Could you check a few things on this model? Use its own coordinates, in mm. A direction names the side the tool comes from. Coordinates: 2 decimals unless noted, no trailing zeros. Order: outer loops, then holes, each group sorted by start corner. A loop starts at its lowest first (then second) coordinate and runs counter-clockwise, first axis right, second up. Notation, with made-up numbers: (56.5, 16.25) - (109.5, 16.25) arc R19 cw to (109.5, 38.25) - close; hole circle Ø4 at (8, -33.75). An arc over 180 degrees is marked (long way). One line per item, written item: value. Start each with the question number.
from build123d import *

# Parameters (mm, degrees)
SKETCH1_W               = 28
SKETCH1_H               = 16
BOSS_EXTRUDE1_DEPTH     = 3
BOSS_EXTRU_1_DEPTH      = 5
BOSS_EXTRU_1_DEPTH_BACK = 18
ESQUISSE8_W             = 11.84
ESQUISSE8_H             = 2.37
ENL_V_MAT_EXTRU_4_DEPTH = 10
ESQUISSE9_W             = 22.6
ESQUISSE9_H             = 11.84
ENL_V_MAT_EXTRU_5_DEPTH = 1
ESQUISSE10_R            = 1.05
ENL_V_MAT_EXTRU_6_DEPTH = 52.879282956
CONG_3_R                = 1
CONG_4_R                = 5
CONG_5_R                = 2.5


with BuildPart() as part:
    # Sketch1 → Boss-Extrude1 (new body)
    with BuildSketch(Plane(origin=(0, 0, 0), x_dir=(1, 0, 0), z_dir=(0, 1, 0))):
        with Locations((14, 8)):
            Rectangle(SKETCH1_W, SKETCH1_H)
    extrude(amount=BOSS_EXTRUDE1_DEPTH)

    # Esquisse1 → Boss.-Extru.1 (add, two sides: drawn at the far end of the back side and taken through both)
    with BuildSketch(Plane.XY.offset(-BOSS_EXTRU_1_DEPTH_BACK)):
        Polygon((32.369048105, 3), (33.869048105, 3.9), (48.5, 3.9), (48.5, 0.9), (34.7, 0.9), (33.2, 0), (28, 0), (28, 3), align=None)
    extrude(amount=BOSS_EXTRU_1_DEPTH + BOSS_EXTRU_1_DEPTH_BACK)

    # Esquisse8 → Enlèv. mat.-Extru.4 (cut)
    with BuildSketch(Plane(origin=(0, 3.9, 0), x_dir=(1, 0, 0), z_dir=(0, 1, 0))):
        with Locations((41.52, 12.315)):
            Rectangle(ESQUISSE8_W, ESQUISSE8_H)
    extrude(amount=-ENL_V_MAT_EXTRU_4_DEPTH, mode=Mode.SUBTRACT)

    # Esquisse9 → Enlèv. mat.-Extru.5 (cut)
    with BuildSketch(Plane.XZ):
        with Locations((15.8, -8)):
            Rectangle(ESQUISSE9_W, ESQUISSE9_H)
    extrude(amount=-ENL_V_MAT_EXTRU_5_DEPTH, mode=Mode.SUBTRACT)

    # Esquisse10 → Enlèv. mat.-Extru.6 (cut, through all)
    with BuildSketch(Plane.XZ):
        with Locations(Location((31.11, 0, 0), (0, 0, 270))):
            Circle(ESQUISSE10_R)
        with Locations(Location((31.11, -16, 0), (0, 0, 270))):
            Circle(ESQUISSE10_R)
    extrude(amount=-ENL_V_MAT_EXTRU_6_DEPTH, mode=Mode.SUBTRACT)

    # Congé3
    cong_3_edges = [part.edges().sort_by_distance(p)[0] for p in [
        (28, 1.5, -16),
    ]]
    fillet(cong_3_edges, radius=CONG_3_R)
    cong_3_2_edges = [part.edges().sort_by_distance(p)[0] for p in [
        (28, 1.5, -18),
    ]]
    fillet(cong_3_2_edges, radius=CONG_3_R - 0.0001)  # a hair under: the kernel refuses the full size

    # Congé4
    cong_4_edges = [part.edges().sort_by_distance(p)[0] for p in [
        (48.5, 2.4, -18),
        (48.5, 2.4, 5),
        (0, 1.5, 0),
        (0, 1.5, -16),
    ]]
    fillet(cong_4_edges, radius=CONG_4_R)

    # Congé5
    cong_5_edges = [part.edges().sort_by_distance(p)[0] for p in [
        (28, 1.5, 0),
    ]]
    fillet(cong_5_edges, radius=CONG_5_R)
    cong_5_2_edges = [part.edges().sort_by_distance(p)[0] for p in [
        (28, 1.5, 5),
    ]]
    fillet(cong_5_2_edges, radius=CONG_5_R - 0.0001)  # a hair under: the kernel refuses the full size


solid = part.part
Q1. I want a section at A-A on x = 42. Please give me the cut outline in (y, z), then the cut area to 3 significant figures.
Q2. I want a section at C-C on z = -0.5. Please give me the cut outline in (x, y).
Q3. We'd pull the mould along Z, two halves only. Please class faces 1 (the flat face through (47.44, 2, -12)), 2 (the flat face through (37, 2, 5)), 3 (the cylindrical face through (2, 2, -15)), 4 (the cylindrical face through (32.15, 1.48, -15.86)): +Z half, -Z half, draft (parallel to the pull), parting line (faces both ways), or undercut.
Q4. I'm going to push flat-ended pins straight in: pin 1 (1 mm diameter, centred on x = 7.5, z = -9.5, fed in from -Y); pin 2 (6 mm diameter, centred on x = 10, z = -1, fed in from -Y); pin 3 (3 mm diameter, centred on x = 32, z = 1.5, fed in from +Y); pin 4 (1.1 mm diameter, centred on x = 10.5, y = 0.5, fed in from +Z). Where does each tip first touch, or does it pass through?
Q5. I want a section at D-D on y = 1.5. State how many separate pieces and enclosed holes the cut face has, then the cut area to 3 significant figures.
Q6. I want a section at B-B on x = 31.11. Please give me the cut outline in (y, z), then the cut area to 3 significant figures.
Q7. If I drill on L1, parallel to Z at x = 36.5, y = 2.2; L2, parallel to Y at x = 41, z = 0.75; L3, parallel to Z at x = 16, y = 2.45, over which ranges is the centre line in solid material (lowest first)?
Q8. Which directions (+Z, -Z, +X, -X, +Y, -Y) give clear straight access to the entire face, cutting with the end or side of a thin tool? Please do faces 5 (the flat face through (27.1, 0.5, -8.1)), 6 (the flat face through (42, 0.9, -7)), 7 (the flat face through (16, 3, -7)), 8 (the flat face through (16, 1, -16)).
Values follow:
1. outline: (0.9, -18) - (3.9, -18) - (3.9, -13.5) - (0.9, -13.5) - close; (0.9, -11.13) - (3.9, -11.13) - (3.9, 5) - (0.9, 5) - close
1. area: 61.9 mm^2
2. outline: (2.82, 0) - (30.19, 0) - (30.19, 3) - (2.82, 3) - close; (32.03, 0) - (33.2, 0) - (34.7, 0.9) - (48.5, 0.9) - (48.5, 3.9) - (33.87, 3.9) - (32.37, 3) - (32.03, 3) - close
3. face 1: undercut
3. face 2: +Z half
3. face 3: -Z half
3. face 4: undercut
4. pin 1: stops at y = 1
4. pin 2: stops at y = 0
4. pin 3: stops at y = 3.68
4. pin 4: stops at z = 0
5. separate pieces: 1
5. enclosed holes: 3
5. area: 863 mm^2
6. outline: (0, -18) - (3, -18) - (3, -17.05) - (0, -17.05) - close; (0, -14.95) - (3, -14.95) - (3, -1.05) - (0, -1.05) - close; (0, 1.05) - (3, 1.05) - (3, 5) - (0, 5) - close
6. area: 56.4 mm^2
7. L1: z = -18 to -13.5, -11.13 to 5
7. L2: y = 0.9 to 3.9
7. L3: z = -16 to 0
8. face 5: -Y
8. face 6: +Z, -Z, +X, -Y
8. face 7: +Z, -Z, -X, +Y
8. face 8: -Z, -X, +Y, -Y
